Geometry check sheet. Reference: the model listing, model coordinates, mm. Coordinates: 2 decimals unless noted, no trailing zeros. Write each loop counter-clockwise with the first axis right and the second up, starting at its lowest first coordinate (ties: lowest second). Pieces come first, ordered by that corner, then holes.
from build123d import *

# Parameters (mm, degrees)
SKETCH_1_R      = 5
SKETCH_1_R_2    = 1.5
EXTRUDE_1_DEPTH = 4
CHAMFER_1_SIZE  = 0.5


with BuildPart() as part:
    # 草图1 → 凸台-拉伸1 (new body)
    with BuildSketch(Plane(origin=(0, 0, 0), x_dir=(1, 0, 0), z_dir=(0, 1, 0))):
        with Locations(Location((0, 0, 0), (0, 0, 270))):
            Circle(SKETCH_1_R)
        with Locations(Location((0, 0, 0), (0, 0, 270))):
            Circle(SKETCH_1_R_2, mode=Mode.SUBTRACT)
    extrude(amount=EXTRUDE_1_DEPTH)

    # 倒角1
    chamfer_1_edges = [part.edges().sort_by_distance(p)[0] for p in [
        (0, 0, -5),
        (0, 4, -5),
        (0, 4, -1.5),
    ]]
    chamfer(chamfer_1_edges, length=CHAMFER_1_SIZE)


solid = part.part
1. Sectioned sample at B-B, the plane z = 0. Record the boundary of the cut face in (x, y).
Computed values:
outline: (-5, 0.5) - (-4.5, 0) - (-1.5, 0) - (-1.5, 3.5) - (-2, 4) - (-4.5, 4) - (-5, 3.5) - close; (1.5, 0) - (4.5, 0) - (5, 0.5) - (5, 3.5) - (4.5, 4) - (2, 4) - (1.5, 3.5) - close
2. Sectioned sample at D-D, the plane y = 3.65. Record the boundary of the cut face in (x, z).
Computed values:
outline: circle Ø9.7 at (0, 0); hole circle Ø3.3 at (0, 0)
3. Thickness scan on line 1 along X through (y, z) = (1.4, 0); line 2 along Z through (x, y) = (0.25, 0.55); line 3 along X through (y, z) = (1.8, -0.75). Record the ranges inside material, lowest first.
Computed values:
line 1: x = -5 to -1.5, 1.5 to 5
line 2: z = -4.99 to -1.48, 1.48 to 4.99
line 3: x = -4.94 to -1.3, 1.3 to 4.94
4. Gauge pin test, flat ends, axial feed: pin 1 Ø1.5 at (x, y) = (-2, 2) entering from +Z; pin 2 Ø1 at (y, z) = (2, -2) entering from -X; pin 3 Ø1.5 at (y, z) = (1, 2.5) entering from -X. Record the tip position at first contact, or that the pin passes through.
Computed values:
pin 1: stops at z = 4.84
pin 2: stops at x = -4.77
pin 3: stops at x = -4.68
5. Draft check along Z on faces 1 (the flat face through (-2, 4, 1)), 2 (the cylindrical face through (0.45, 1.73, 1.43)), 3 (the cylindrical face through (-4.88, 1.98, -1.08)). Enter one of: released by +Z, released by -Z, zero draft, split by the parting line, or undercut.
Computed values:
face 1: zero draft
face 2: undercut
face 3: split by the parting line
6. Sectioned sample at A-A, the plane x = 0. Record the boundary of the cut face in (y, z).
Computed values:
outline: (0, -4.5) - (0.5, -5) - (3.5, -5) - (4, -4.5) - (4, -2) - (3.5, -1.5) - (0, -1.5) - close; (0, 1.5) - (3.5, 1.5) - (4, 2) - (4, 4.5) - (3.5, 5) - (0.5, 5) - (0, 4.5) - close
7. Sectioned sample at C-C, the plane y = 1.8. Record the boundary of the cut face in (x, z).
Computed values:
outline: circle Ø10 at (0, 0); hole circle Ø3 at (0, 0)
